CAD build for the part. Positions are in the model's coordinates, mm. Give positions to 0.01 mm unless a question says otherwise; leave off trailing zeros. Order: outer loops, then holes, each group sorted by start corner. A loop starts at its lowest first (then second) coordinate and runs counter-clockwise, first axis right, second up.
Item 1: Band-saw the part on C-C on x = 54. Give the cut face in (y, z).
Item 2: Band-saw the part on B-B on y = 1.25. Give the cut face in (x, z).
Item 3: Band-saw the part on D-D on z = -10.5. Give the cut face in (x, y).
Item 4: Band-saw the part on A-A on z = 0. Give the cut face in (x, y).
Item 5: Flat gauge pins, fed straight in: P1, Ø3, axis at y = 1.5, z = -21.5, coming from the +X side; P2, Ø2.5, axis at x = 97.01, z = 0, coming from the -Y side. Where does each tip first touch, or does it go through?
Item 6: Wall check: L1, parallel to X at y = 3, z = 0.5; L2, parallel to X at y = 3.75, z = -1; L3, parallel to Z at x = 35.5, y = 8. Give the ranges that are in metal, low to high.
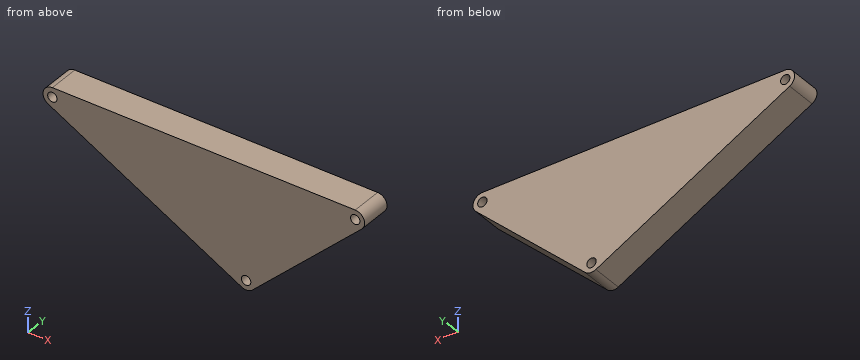
Autodesk Inventor part; units mm, degrees
ref_plane "YZ Plane" through (0, 0, 0) normal (1, 0, 0) x (0, 1, 0)
ref_plane "XZ Plane" through (0, 0, 0) normal (0, 1, 0) x (-1, 0, 0)
ref_plane "XY Plane" through (0, 0, 0) normal (0, 0, 1) x (1, 0, 0)
sketch "草圖2" plane through (0, 0, 0) normal (0, 1, 0) x (-1, 0, 0)
  line L0 (-62.0601, -33.0641) -> (0, 0) construction
  line L1 (0, 0) -> (-97.0141, 0) construction
  arc A0 (-97.0141, 3) -> (-99.0756, -2.1794) centre (-97.0141, 0) ccw
  arc A1 (1.4106, -2.6477) -> (0, 3) centre (0, 0) ccw
  line L2 (-97.0141, 3) -> (0, 3)
  line L3 (-99.0756, -2.1794) -> (-64.1217, -35.2435)
  line L4 (-97.0141, 0) -> (-62.0601, -33.0641) construction
  arc A2 (-64.1217, -35.2435) -> (-60.6495, -35.7117) centre (-62.0601, -33.0641) ccw
  line L5 (1.4106, -2.6477) -> (-60.6495, -35.7117)
  circle A3 centre (-97.0141, 0) radius 1.5
  circle A4 centre (0, 0) radius 1.5
  circle A5 centre (-62.0601, -33.0641) radius 1.5
  dimension "d11" = 6
  dimension "hole" = 3
  dimension "center_distance1" = 97.0141
  dimension "center_distance3" = 48.1146
  dimension "center_distance2" = 70.3185
extrude "擠出2" add sketch "草圖2" along normal blind 10
equation "\"d11\" = 2 * hole"
properties part number "ternary_link"
The answers:
1. outline: (0, -32.17) - (10, -32.17) - (10, 3) - (0, 3) - close
2. outline: (-1.41, -2.65) - (60.65, -35.71) arc R3 ccw to (64.12, -35.24) - (99.08, -2.18) arc R3 ccw to (97.01, 3) - (0, 3) arc R3 ccw to start; hole circle Ø3 at (0, 0); hole circle Ø3 at (62.06, -33.06); hole circle Ø3 at (97.01, 0)
3. outline: (13.33, 0) - (90.28, 0) - (90.28, 10) - (13.33, 10) - close
4. outline: (-3, 0) - (-1.5, 0) - (-1.5, 10) - (-3, 10) - close; (1.5, 0) - (95.51, 0) - (95.51, 10) - (1.5, 10) - close; (98.51, 0) - (100.01, 0) - (100.01, 10) - (98.51, 10) - close
5. P1: stops at x = 80.24
5. P2: passes through
6. L1: x = -2.96 to -1.41, 1.41 to 95.6, 98.43 to 99.97
6. L2: x = -2.83 to -1.12, 1.12 to 95.9, 98.13 to 99.84
6. L3: z = -22.31 to 3
